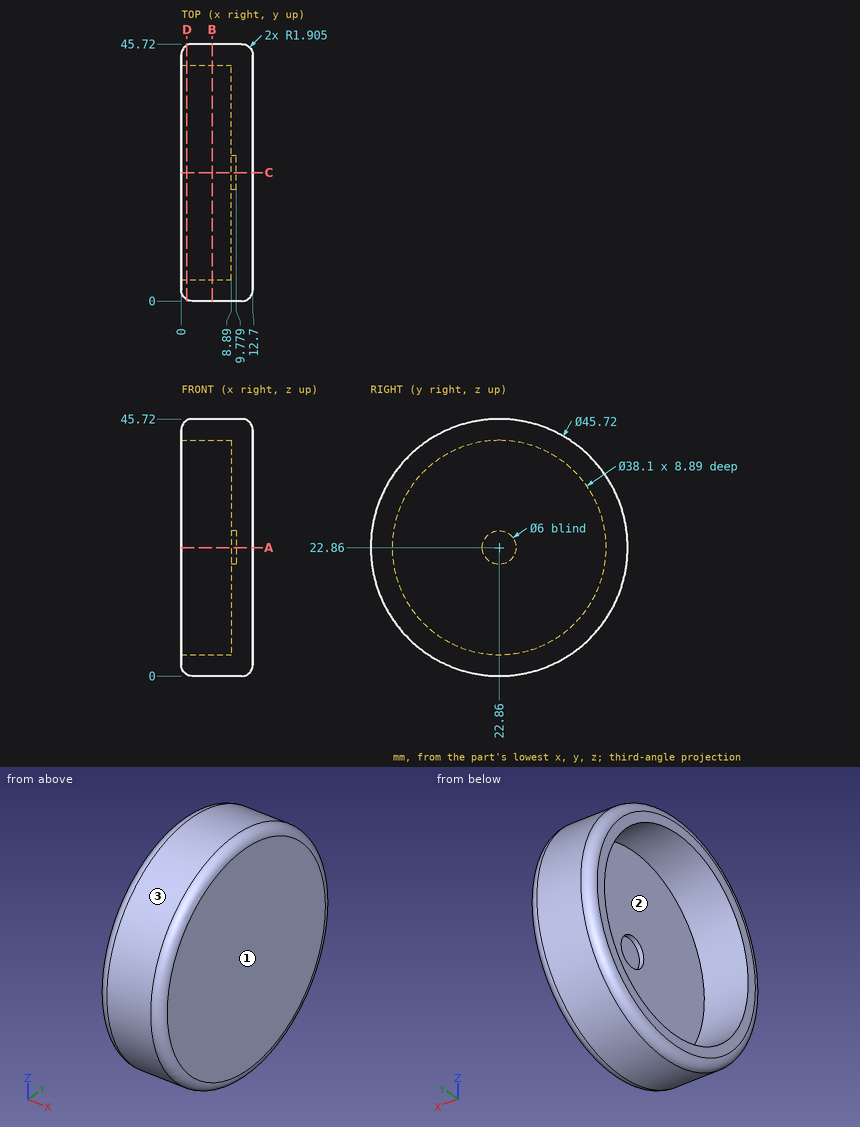
Geometry: see drawing. Coordinates: mm, zero at the bounding-box minimum. Coordinates: 2 decimals unless noted, no trailing zeros. Loops run counter-clockwise (first coordinate to the right, second up) from the corner with the lowest first, then second, coordinate; pieces in that order, holes last. Notation, with made-up numbers: M 38.5,58 L 75.5,58 A20 cw 75.5,86 Z; hole C 68.25,9 d4. An arc over 180 degrees is marked long. Answer in a Markdown table with one row per item.
Q1. Section B-B on x = 5.5. Return the cut outline in (y, z).
Answers below:
| item | result |
|---|---|
| outline | C 22.86,22.86 d45.72; hole C 22.86,22.86 d38.1 |
Q2. Section A-A on z = 22.86. Return the cut outline in (x, y) (3 decimals).
Answers below:
| item | result |
|---|---|
| outline | M 0,1.905 A1.905 ccw 1.905,0 L 10.795,0 A1.905 ccw 12.7,1.905 L 12.7,43.815 A1.905 ccw 10.795,45.72 L 1.905,45.72 A1.905 ccw 0,43.815 L 0,41.91 L 8.89,41.91 L 8.89,25.86 L 9.779,25.86 L 9.779,19.86 L 8.89,19.86 L 8.89,3.81 L 0,3.81 Z |
Q3. Section D-D on x = 1. Return the cut outline in (y, z), plus the area to 3 significant figures.
Answers below:
| item | result |
|---|---|
| outline | C 22.86,22.86 d45.26; hole C 22.86,22.86 d38.1 |
| area | 469 mm^2 |
Q4. Ray query, probe 1 along Y at (x, z) = (2.25, 22.86); probe 2 along Z at (x, y) = (9.4, 22.86). Return the intervals inside material, ascending. Write a range as from..to.
Answers below:
| item | result |
|---|---|
| probe 1 | y = 0..3.81, 41.91..45.72 |
| probe 2 | z = 0..19.86, 25.86..45.72 |
Q5. First-contact query: pin 1 (1 mm diameter, centred on x = 5, z = 35.5, fed in from -Y); pin 2 (1.8 mm diameter, centred on y = 22.5, z = 22, fed in from -X); pin 3 (1 mm diameter, centred on x = 3.5, z = 6, fed in from +Y). Flat tips, straight axial feed; report the tip coordinate or a pass-through.
Answers below:
| item | result |
|---|---|
| pin 1 | stops at y = 3.49 |
| pin 2 | stops at x = 9.78 |
| pin 3 | stops at y = 38.83 |
Q6. Draft query along Y for the marked faces 1, 2 and 3. Return one class per face: pulls with the +Y half, pulls with the -Y half, needs draft (parallel to the pull), parting line crosses it, or undercut.
Answers below:
| item | result |
|---|---|
| face 1 | needs draft |
| face 2 | undercut |
| face 3 | parting line crosses it |
